```python
from build123d import *

# Parameters (mm, degrees)
F1_DEPTH      = 9.525
F2_R          = 2.54
F3_DEPTH      = 25.4
F3_DEPTH_BACK = 25.4


with BuildPart() as f1:
    # F0 (on Top) → F1 (new body)
    with BuildSketch(Plane.XY):
        with BuildLine():
            ThreePointArc((-20.955, 0), (-14.8174225998, 14.8174225998), (0, 20.955))
            ThreePointArc((0, 20.955), (14.8174225998, 14.8174225998), (20.955, 0))
            Line((20.955, 0), (20.955, -20.955))
            Line((20.955, -20.955), (36.83, -20.955))
            Line((36.83, -20.955), (36.83, -14.605))
            Line((36.83, -14.605), (30.48, -14.605))
            ThreePointArc((30.48, -14.605), (25.9898719395, -12.7451280605), (24.13, -8.255))
            Line((24.13, -8.255), (24.13, 0))
            ThreePointArc((24.13, 0), (17.06248663, 17.06248663), (0, 24.13))
            ThreePointArc((0, 24.13), (-17.06248663, 17.06248663), (-24.13, 0))
            Line((-24.13, 0), (-24.13, -8.255))
            ThreePointArc((-24.13, -8.255), (-25.9898719395, -12.7451280605), (-30.48, -14.605))
            Line((-30.48, -14.605), (-36.83, -14.605))
            Line((-36.83, -14.605), (-36.83, -20.955))
            Line((-36.83, -20.955), (-20.955, -20.955))
            Line((-20.955, -20.955), (-20.955, 0))
        make_face()
    extrude(amount=F1_DEPTH)

    # F2 (on face) → F3 (cut, two sides)
    with BuildSketch(Plane(origin=(0, -14.605, 0), x_dir=(-1, 0, 0), z_dir=(0, 1, 0))) as f3_sk:
        with Locations((-31.115, 4.7625)):
            Circle(F2_R)
        with BuildLine():
            Line((30.48, 2.3031555752), (30.48, 7.2218444248))
            ThreePointArc((30.48, 7.2218444248), (28.575, 4.7625), (30.48, 2.3031555752))
        make_face()
        with BuildLine():
            ThreePointArc((30.48, 2.3031555752), (32.6704259867, 2.7544536858), (33.655, 4.7625))
            ThreePointArc((33.655, 4.7625), (32.6704259867, 6.7705463142), (30.48, 7.2218444248))
            Line((30.48, 7.2218444248), (30.48, 2.3031555752))
        make_face()
    extrude(amount=-F3_DEPTH, mode=Mode.SUBTRACT)
    extrude(f3_sk.sketch, amount=F3_DEPTH_BACK, mode=Mode.SUBTRACT)


solid = f1.part
```
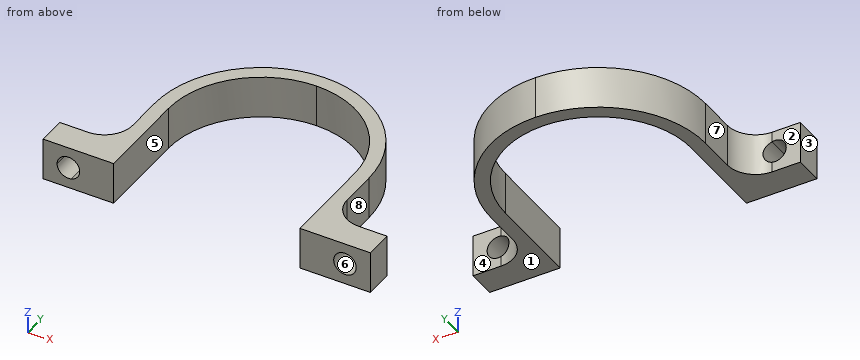
The listing builds one solid part. Answer for the finished solid, in the listing's coordinates (mm). Face numbers are marked on the shaded views. A direction names the side the tool comes from. Give positions to 0.01 mm unless a question says otherwise; leave off trailing zeros. Order: outer loops, then holes, each group sorted by start corner. A loop starts at its lowest first (then second) coordinate and runs counter-clockwise, first axis right, second up.
1) For the marked faces 1, 2, 3, 4 and 5, determine the directions among +Z, -Z, +X, -X, +Y, -Y from which every point of the face is accessible in a straight line to the end or side of a thin tool.
Reported:
face 1: -Z, +X, -X, +Y, -Y
face 2: +Z, -Z, -X, +Y
face 3: +Z, -Z, -X, +Y, -Y
face 4: +Z, -Z, +X, +Y
face 5: +Z, -Z, -Y
2) Consider line 1 along X through (y, z) = (-6, 0.5) (3 decimals); line 2 along X through (y, z) = (-17, 9.25) (3 decimals); line 3 along Y through (x, z) = (33.5, 9.25) (3 decimals). Determine where each line is inside the solid, lowest interval first.
Reported:
line 1: x = -24.13 to -20.955, 20.955 to 24.13
line 2: x = -36.83 to -20.955, 20.955 to 36.83
line 3: y = -20.955 to -14.605
3) Given P1, Ø1, axis at x = 15.5, z = 2.5, coming from the +Y side; P2, Ø3, axis at y = 10.5, z = 6.5, coming from the +X side; P3, Ø5, axis at x = 34, z = 4, coming from the +Y side (3 decimals), each flat-ended and moving along its own axis, determine where each tip first touches the part or whether it passes through.
Reported:
P1: stops at y = 18.9
P2: stops at x = 22.39
P3: stops at y = -14.605
4) Find section B-B on z = 6.5. Write down the section's boundary in (x, y) (3 decimals).
Reported:
outline: (-36.83, -20.955) - (-32.968, -20.955) - (-32.968, -14.605) - (-36.83, -14.605) - close; (-29.262, -20.955) - (-20.955, -20.955) - (-20.955, 0) arc R20.955 cw to (20.955, 0) - (20.955, -20.955) - (29.262, -20.955) - (29.262, -14.487) arc R6.35 cw to (24.13, -8.255) - (24.13, 0) arc R24.13 ccw to (-24.13, 0) - (-24.13, -8.255) arc R6.35 cw to (-29.262, -14.487) - close; (32.968, -20.955) - (36.83, -20.955) - (36.83, -14.605) - (32.968, -14.605) - close
5) Find section C-C on x = -32. Write down the section's boundary in (y, z) (3 decimals), then the cut area to 3 significant figures.
Reported:
outline: (-20.955, 0) - (-14.605, 0) - (-14.605, 2.382) - (-20.955, 2.382) - close; (-20.955, 7.143) - (-14.605, 7.143) - (-14.605, 9.525) - (-20.955, 9.525) - close
area: 30.2 mm2
6) Determine the mould class of the marked faces 6, 7 and 8 for opening direction X: pulls with the +X half, pulls with the -X half, needs draft (parallel to the pull), parting line crosses it, or undercut.
Reported:
face 6: undercut
face 7: pulls with the -X half
face 8: pulls with the +X half
7) Find section A-A on y = -16. Write down the section's boundary in (x, z) (1 decimal).
Reported:
outline: (-36.8, 0) - (-21, 0) - (-21, 9.5) - (-36.8, 9.5) - close; (21, 0) - (36.8, 0) - (36.8, 9.5) - (21, 9.5) - close; hole circle Ø5.1 at (-31.1, 4.8); hole circle Ø5.1 at (31.1, 4.8)
8) Find section D-D on y = 15. Write down the section's boundary in (x, z) (3 decimals).
Reported:
outline: (-18.901, 0) - (-14.633, 0) - (-14.633, 9.525) - (-18.901, 9.525) - close; (14.633, 0) - (18.901, 0) - (18.901, 9.525) - (14.633, 9.525) - close
